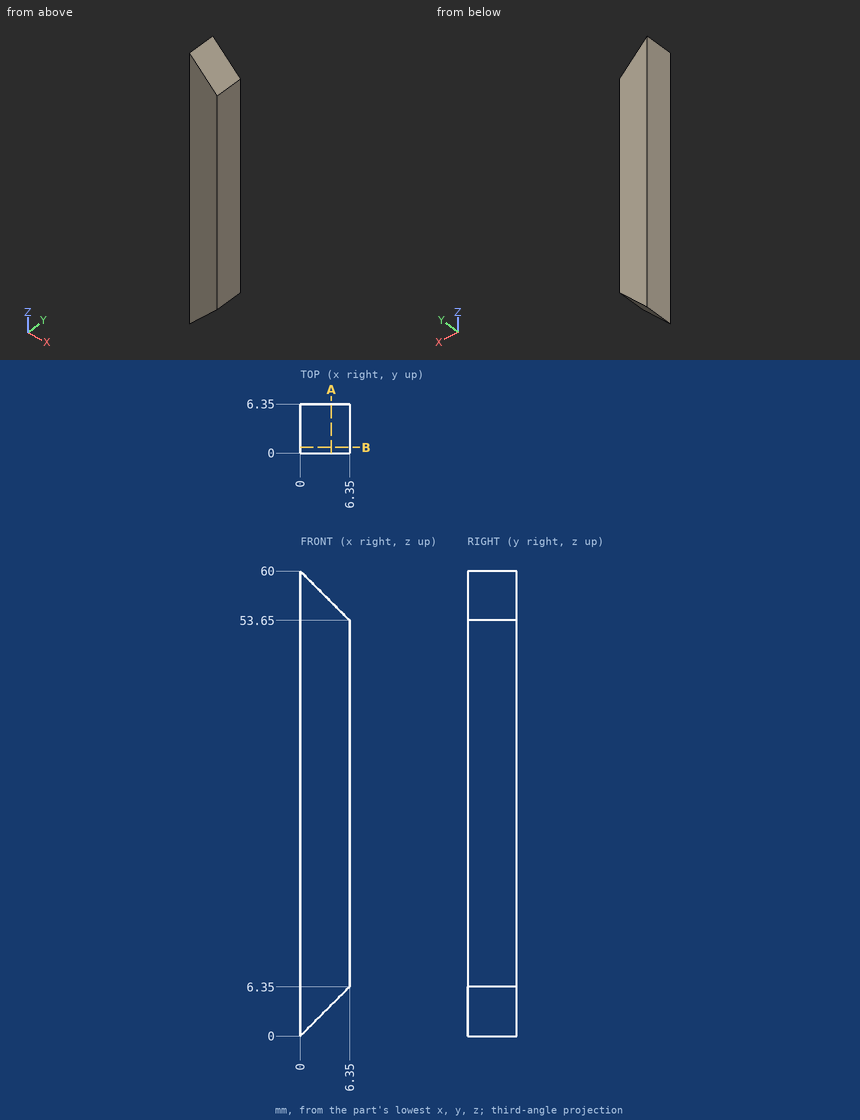
Design review of the part shown in the three views and the two pictorial views. Dimensions are in mm from the part's minimum x, y and z. Give positions to 0.01 mm unless a question says otherwise; leave off trailing zeros. Write each loop counter-clockwise with the first axis right and the second up, starting at its lowest first coordinate (ties: lowest second). Pieces come first, ordered by that corner, then holes. Notation, with made-up numbers: M 56,49.5 L 62,49.5 A20 cw 62,61.5 Z; hole C 47,67 d1. An arc over 180 degrees is marked long. One line per question, with ' | ' between items. Start each with the question number.
Item 1: We need section B-B on y = 0.75. Write out the cut boundary in (x, z), plus the area to 3 significant figures.
Item 2: We need section A-A on x = 4. Write out the cut boundary in (y, z), plus the area to 3 significant figures.
Item 3: Wall thickness on line 1 (X direction, y = 3.5, z = 54.5); line 2 (Z direction, x = 6.25, y = 1.25); line 3 (Z direction, x = 3, y = 2.5): over which ranges is each line inside the solid? List them lowest first. Write a range as from..to.
Results found:
1) outline: M 0,0 L 6.35,6.35 L 6.35,53.65 L 0,60 Z | area: 341 mm2
2) outline: M 0,4 L 6.35,4 L 6.35,56 L 0,56 Z | area: 330 mm2
3) line 1: x = 0..5.5 | line 2: z = 6.25..53.75 | line 3: z = 3..57
